Can you work these out from the model? Positions are in its coordinate system, mm. Round coordinates to 2 decimals unless told otherwise and drop trailing zeros. Loops run counter-clockwise (first coordinate to the right, second up) from the corner with the lowest first, then second, coordinate; pieces in that order, holes last. Notation, with made-up numbers: (-33.5, 78) - (-7.5, 78) arc R16 ccw to (-7.5, 84) - close; hole circle Ø1 at (49.25, -24). An arc over 180 degrees is marked (long way). Answer as CSV lines item,"result".
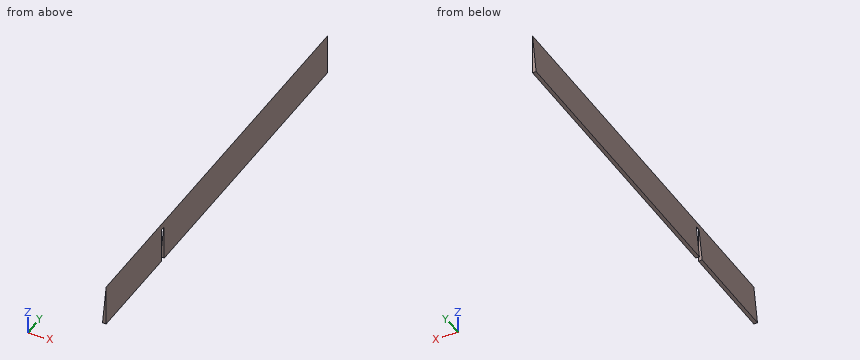
```python
from build123d import *

# Parameters (mm, degrees)
F0_R     = 200
F1_DEPTH = 2000
F3_R     = 377.245837
F3_W     = 300
F3_H     = 60
F4_DEPTH = 25
F6_DEPTH = 2000


with BuildPart() as f1:
    # F0 (on Front) → F1 (new body)
    with BuildSketch(Plane.XZ):
        Circle(F0_R)
    extrude(amount=F1_DEPTH)

    # F3 (on offset) → F4 (cut)
    with BuildSketch(Plane.XZ.offset(1500)):
        Circle(F3_R)
        Rectangle(F3_W, F3_H, mode=Mode.SUBTRACT)
    extrude(amount=-F4_DEPTH, mode=Mode.SUBTRACT)

    # F5 (on face) → F6 (intersect)
    with BuildSketch(Plane.XZ.offset(2000)):
        with BuildLine():
            Line((0, -200), (0, 0))
            Line((0, 0), (-17.431149, -199.23894))
            ThreePointArc((-17.431149, -199.23894), (-8.723877, -199.809644), (0, -200))
        make_face()
    extrude(amount=-F6_DEPTH, mode=Mode.INTERSECT)


solid = f1.part
```
Q1. If I drill on line 1 along Y through (x, z) = (-8.5, -135); line 2 along X through (y, z) = (-1004, -26); line 3 along X through (y, z) = (-835, -104.5), over which ranges is the centre line in solid material (lowest first)? Write a range as [from, to].
Checks:
line 1,"[-2000, -1500], [-1475, 0]"
line 2,"[-2.27, 0]"
line 3,"[-9.14, 0]"
Q2. Imagine slicing it at C-C (y = -457). Write out the boundary of the cut face in (x, z), then the cut area to 3 significant figures.
Checks:
outline,"(-17.43, -199.24) arc R200 ccw to (0, -200) - (0, 0) - close"
area,"1,750 mm²"
Q3. I'm going to push flat-ended pins straight in: pin 1 Ø8 at (y, z) = (-1304, -142) entering from -X; pin 2 Ø3 at (x, y) = (-9.5, -1123) entering from -Z; pin 3 Ø3 at (x, y) = (-2, -1482) entering from -Z; pin 4 Ø2 at (x, z) = (-4.5, -25.5) entering from -Y. Where does each tip first touch, or does it pass through?
Checks:
pin 1,"x = -12.77"
pin 2,"z = -199.84"
pin 3,"z = -30"
pin 4,"through"
Q4. Imagine slicing it at A-A (z = -113). Write out the boundary of the cut face in (x, y).
Checks:
outline,"(-9.89, -2000) - (0, -2000) - (0, -1500) - (-9.89, -1500) - close; (-9.89, -1475) - (0, -1475) - (0, 0) - (-9.89, 0) - close"
Q5. Imagine slicing it at B-B (x = -10). Write out the boundary of the cut face in (y, z), then the cut area to 3 significant figures.
Checks:
outline,"(-2000, -199.75) - (-1500, -199.75) - (-1500, -114.3) - (-2000, -114.3) - close; (-1475, -199.75) - (0, -199.75) - (0, -114.3) - (-1475, -114.3) - close"
area,"169,000 mm²"
